```python
from build123d import *

# Parameters (mm, degrees)
BOSS_EXTRUDE1_DEPTH  = 4.7625
M4_CLEARANCE_HOLE1_D = 4.5


with BuildPart() as part:
    # Sketch1 → Boss-Extrude1 (new body)
    with BuildSketch(Plane.XY):
        with BuildLine():
            Line((-94, 144.919812433), (-94, 129.845444943))
            ThreePointArc((-94, 129.845444943), (-95.255453966, 126.532081848), (-98.39135, 124.882628688))
            ThreePointArc((-98.39135, 124.882628688), (-102.7827, 119.919812433), (-98.39135, 114.956996179))
            ThreePointArc((-98.39135, 114.956996179), (-95.255453966, 113.307543019), (-94, 109.994179924))
            Line((-94, 109.994179924), (-94, 60.005820076))
            ThreePointArc((-94, 60.005820076), (-95.255453966, 56.692456981), (-98.39135, 55.043003821))
            ThreePointArc((-98.39135, 55.043003821), (-102.7827, 50.080187567), (-98.39135, 45.117371312))
            ThreePointArc((-98.39135, 45.117371312), (-95.255453966, 43.467918152), (-94, 40.154555057))
            Line((-94, 40.154555057), (-94, 25.080187567))
            ThreePointArc((-94, 25.080187567), (-93.285154037, 22.412797084), (-91.332218978, 20.460357228))
            Line((-91.332218978, 20.460357228), (-70.871308953, 8.651857213))
            ThreePointArc((-70.871308953, 8.651857213), (-68.590749548, 5.788703611), (-68.871909852, 2.13910793))
            ThreePointArc((-68.871909852, 2.13910793), (-66.715485478, -4.460545697), (-60.042693242, -2.542359614))
            Line((-60.042693242, -2.542359614), (-59.97854154, -2.431202209))
            ThreePointArc((-59.97854154, -2.431202209), (-57.893008537, -0.462819662), (-55.068956864, 0.035888574))
            ThreePointArc((-55.068956864, 0.035888574), (-54.760620401, 0.008979702), (-54.451242271, 0))
            Line((-54.451242271, 0), (-15.925632509, 0))
            ThreePointArc((-15.925632509, 0), (-12.612269414, -1.255453966), (-10.962816255, -4.39135))
            ThreePointArc((-10.962816255, -4.39135), (-5.69510762, -8.773395406), (-1, -3.7827))
            Line((-1, -3.7827), (-0.126827546, 4.177751308))
            ThreePointArc((-0.126827546, 4.177751308), (-0.031801689, 4.752408162), (0, 5.334))
            Line((0, 5.334), (0, 40.154555057))
            ThreePointArc((0, 40.154555057), (1.255453966, 43.467918152), (4.39135, 45.117371312))
            ThreePointArc((4.39135, 45.117371312), (8.7827, 50.080187567), (4.39135, 55.043003821))
            ThreePointArc((4.39135, 55.043003821), (1.255453966, 56.692456981), (0, 60.005820076))
            Line((0, 60.005820076), (0, 109.994179924))
            ThreePointArc((0, 109.994179924), (1.255453966, 113.307543019), (4.39135, 114.956996179))
            ThreePointArc((4.39135, 114.956996179), (8.7827, 119.919812433), (4.39135, 124.882628688))
            ThreePointArc((4.39135, 124.882628688), (1.255453966, 126.532081848), (0, 129.845444943))
            Line((0, 129.845444943), (0, 164.666))
            ThreePointArc((0, 164.666), (-0.031801689, 165.247591838), (-0.126827546, 165.822248692))
            Line((-0.126827546, 165.822248692), (-1, 173.7827))
            ThreePointArc((-1, 173.7827), (-5.69510762, 178.773395406), (-10.962816255, 174.39135))
            ThreePointArc((-10.962816255, 174.39135), (-12.612269414, 171.255453966), (-15.925632509, 170))
            Line((-15.925632509, 170), (-54.451242271, 170))
            ThreePointArc((-54.451242271, 170), (-54.760620401, 169.991020298), (-55.068956864, 169.964111426))
            ThreePointArc((-55.068956864, 169.964111426), (-57.893008537, 170.462819662), (-59.97854154, 172.431202209))
            Line((-59.97854154, 172.431202209), (-60.042693242, 172.542359614))
            ThreePointArc((-60.042693242, 172.542359614), (-66.715485478, 174.460545697), (-68.871909852, 167.86089207))
            ThreePointArc((-68.871909852, 167.86089207), (-68.590749548, 164.211296389), (-70.871308953, 161.348142787))
            Line((-70.871308953, 161.348142787), (-91.332218978, 149.539642772))
            ThreePointArc((-91.332218978, 149.539642772), (-93.285154037, 147.587202916), (-94, 144.919812433))
        make_face()
    extrude(amount=-BOSS_EXTRUDE1_DEPTH)

    # M4 Clearance Hole1 (through all)
    with Locations(Plane(origin=(0, 0, -4.7625), x_dir=(-1, 0, 0), z_dir=(0, 0, -1))):
        with Locations((6, -3.7827), (-3.7827, 50.080187567), (-3.7827, 119.919812433), (6, 173.7827), (64.373242866, 170.04309173), (97.7827, 119.919812433), (97.7827, 50.080187567), (64.373242866, -0.04309173)):
            Hole(M4_CLEARANCE_HOLE1_D / 2)


solid = part.part
```
For this review, take the finished solid that the model builds, in its own axes (mm). A direction names the side the tool comes from. Give positions to 0.01 mm unless a question says otherwise; leave off trailing zeros. Write each loop counter-clockwise with the first axis right and the second up, starting at its lowest first coordinate (ties: lowest second). Pieces come first, ordered by that corner, then holes. Notation, with made-up numbers: M -30.75,9 L 11.25,9 A23 ccw 11.25,26 Z; hole C 28.25,18 d11. An arc over 180 degrees is marked long. Answer as CSV lines item,"result".
1. For pin 1 (1.4 mm diameter, centred on y = 90.5, z = -2, fed in from +X); pin 2 (2.5 mm diameter, centred on x = -64.37, y = 170.04, fed in from -Z); pin 3 (5 mm diameter, centred on x = -64.37, y = -0.04, fed in from -Z); pin 4 (2 mm diameter, centred on y = 69.5, z = -2, fed in from -X), all flat-tipped, find the tip position at first contact; note any pin that passes through.
Findings:
pin 1,"stops at x = 0"
pin 2,"passes through"
pin 3,"stops at z = -4.76"
pin 4,"stops at x = -94"
2. For faces 1 (the flat face through (-35, 170, -2)), 2 (the flat face through (-35, 0, -2)), 3 (the flat face through (-94, 33, -2)), 4 (the flat face through (0, 85, -2)), list the 3-axis set-ups (+Z, -Z, +X, -X, +Y, -Y) from which the entire face can be reached by the end or side of a thin tool; tool diameter is ignored.
Findings:
face 1,"+Z, -Z, +Y"
face 2,"+Z, -Z, -Y"
face 3,"+Z, -Z, -X, -Y"
face 4,"+Z, -Z, +X"
3. Consider section B-B, the plane x = -35.5. Write out the cut boundary in (y, z), then the cut area to 3 significant figures.
Findings:
outline,"M 0,-4.76 L 170,-4.76 L 170,0 L 0,0 Z"
area,"810 mm2"
4. Wall thickness on line 1 (Y direction, x = -6, z = -3.5); line 2 (Y direction, x = -64.5, z = -2.8); line 3 (Y direction, x = 2, z = -2.8): over which ranges is each line inside the solid? List them lowest first.
Findings:
line 1,"y = -8.78 to -6.03, -1.53 to 171.53, 176.03 to 178.78"
line 2,"y = -5.04 to -2.29, 2.2 to 167.8, 172.29 to 175.04"
line 3,"y = 44.15 to 48.71, 51.45 to 56.01, 113.99 to 118.55, 121.29 to 125.85"
5. Consider section A-A, the plane x = -6. Write out the cut boundary in (y, z), then the cut area to 3 significant figures.
Findings:
outline,"M -8.78,-4.76 L -6.03,-4.76 L -6.03,0 L -8.78,0 Z; M -1.53,-4.76 L 171.53,-4.76 L 171.53,0 L -1.53,0 Z; M 176.03,-4.76 L 178.78,-4.76 L 178.78,0 L 176.03,0 Z"
area,"850 mm2"
6. Draft analysis for pull direction X (two halves, no side actions). For faces 5 (the cylindrical face through (-57.93, -0.48, -2.35)), 6 (the flat face through (-81.245, 14.639, -2.348)), 7 (the flat face through (-48, 86, 0)), state which applies: +X half, -X half, draft (parallel to the pull), parting line (faces both ways), or undercut.
Findings:
face 5,"undercut"
face 6,"-X half"
face 7,"draft"
7. Consider section C-C, the plane y = 158. Write out the cut boundary in (x, z).
Findings:
outline,"M -76.67,-4.76 L 0,-4.76 L 0,0 L -76.67,0 Z"
8. Consider section D-D, the plane z = -2.1. Count the separate pieces of the cut face and the enclosed holes in it, then the cut area to 3 significant figures.
Findings:
separate pieces,"1"
enclosed holes,"8"
area,"15,700 mm2"
